Input: part model. Units: mm. Frame: model coordinates. Face numbers are marked on the shaded views. Round coordinates to 2 decimals unless told otherwise and drop trailing zeros. Order: outer loops, then holes, each group sorted by start corner. A loop starts at its lowest first (then second) coordinate and runs counter-clockwise, first axis right, second up.
Item 1: First-contact query: pin 1 (1.9 mm diameter, centred on y = -9.5, z = 95, fed in from +X). Flat tip, straight axial feed; report the tip coordinate or a pass-through.
Item 2: Cut plane D-D on z = 104. Output: boundary loops of the cut face in (x, y).
Item 3: Cut plane B-B on z = 88.9. Output: boundary loops of the cut face in (x, y).
Item 4: Mould query, pull axis Y, two halves, no side actions, for the marked faces 1, 2 and 3. Classes: released by +Y, released by -Y, zero draft, split by the parting line, or undercut.
Item 5: Cut plane A-A on y = -8.75. Output: boundary loops of the cut face in (x, z), then the cut area to 3 significant figures.
Item 6: Line query: L1, parallel to Z at x = 12.7, y = -1.5; L2, parallel to Z at x = 14.25, y = -1.75; L3, parallel to X at y = -9.25, z = 12.7. Output: solid intervals per line, ascending.
Item 7: Cut plane C-C on x = 22.5. Output: boundary loops of the cut face in (y, z), then the cut area to 3 significant figures.
```python
from build123d import *

# Parameters (mm, degrees)
BOSS_EXTRUDE1_DEPTH                              = 127
CBORE_FOR_1_4_SOCKET_HEAD_CAP_SCREW1_D           = 7.14248
CBORE_FOR_1_4_SOCKET_HEAD_CAP_SCREW1_CBORE_D     = 11.1125
CBORE_FOR_1_4_SOCKET_HEAD_CAP_SCREW1_CBORE_DEPTH = 6.35


with BuildPart() as part:
    # Sketch1 → Boss-Extrude1 (new body)
    with BuildSketch(Plane.XY):
        Polygon((0, 0), (25.4, 0), (21.000590949, -7.62), (21.000590949, -11.43), (25.4, -11.43), (25.4, -17.78), (0, -17.78), (0, -11.43), (4.399409051, -11.43), (4.399409051, -7.62), align=None)
    extrude(amount=BOSS_EXTRUDE1_DEPTH)

    # CBORE for 1/4 Socket Head Cap Screw1 (through all)
    with Locations(Plane(origin=(0, 0, 0), x_dir=(1, 0, 0), z_dir=(0, 1, 0))):
        with Locations((12.7, -12.7), (12.7, -38.1), (12.7, -63.5), (12.7, -88.9), (12.7, -114.3)):
            CounterBoreHole(CBORE_FOR_1_4_SOCKET_HEAD_CAP_SCREW1_D / 2, CBORE_FOR_1_4_SOCKET_HEAD_CAP_SCREW1_CBORE_D / 2, CBORE_FOR_1_4_SOCKET_HEAD_CAP_SCREW1_CBORE_DEPTH)


solid = part.part
```
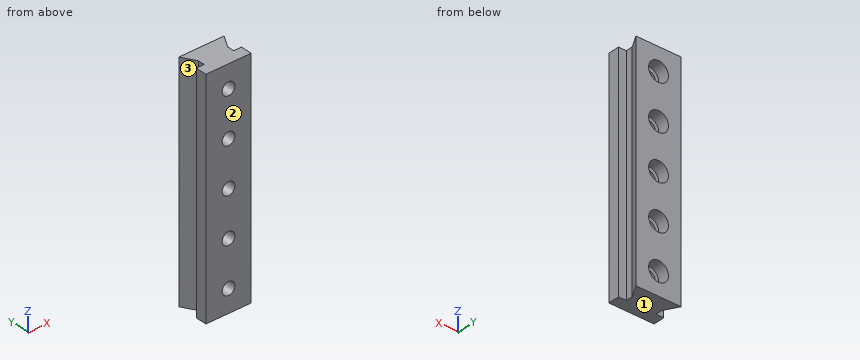
From the geometry:
1. pin 1: stops at x = 21
2. outline: (0, -17.78) - (25.4, -17.78) - (25.4, -11.43) - (21, -11.43) - (21, -7.62) - (25.4, 0) - (0, 0) - (4.4, -7.62) - (4.4, -11.43) - (0, -11.43) - close
3. outline: (0, -17.78) - (9.13, -17.78) - (9.13, -6.35) - (7.14, -6.35) - (7.14, 0) - (0, 0) - (4.4, -7.62) - (4.4, -11.43) - (0, -11.43) - close; (16.27, -17.78) - (25.4, -17.78) - (25.4, -11.43) - (21, -11.43) - (21, -7.62) - (25.4, 0) - (18.26, 0) - (18.26, -6.35) - (16.27, -6.35) - close
4. face 1: zero draft
4. face 2: released by -Y
4. face 3: undercut
5. outline: (4.4, 0) - (21, 0) - (21, 127) - (4.4, 127) - close; hole circle Ø7.14 at (12.7, 12.7); hole circle Ø7.14 at (12.7, 38.1); hole circle Ø7.14 at (12.7, 63.5); hole circle Ø7.14 at (12.7, 88.9); hole circle Ø7.14 at (12.7, 114.3)
5. area: 1,910 mm2
6. L1: z = 0 to 7.14, 18.26 to 32.54, 43.66 to 57.94, 69.06 to 83.34, 94.46 to 108.74, 119.86 to 127
6. L2: z = 0 to 7.36, 18.04 to 32.76, 43.44 to 58.16, 68.84 to 83.56, 94.24 to 108.96, 119.64 to 127
6. L3: x = 4.4 to 9.13, 16.27 to 21
7. outline: (-17.78, 0) - (-11.43, 0) - (-11.43, 127) - (-17.78, 127) - close; (-5.02, 0) - (0, 0) - (0, 127) - (-5.02, 127) - close
7. area: 1,440 mm2
